```python
from build123d import *

# Parameters (mm, degrees)
BOSS_EXTRUDE1_DEPTH = 4.4
SKETCH2_R           = 9.375
BOSS_EXTRUDE2_DEPTH = 0.9
SKETCH3_R           = 7
BOSS_EXTRUDE3_DEPTH = 0.1
SKETCH4_R           = 2.8
BOSS_EXTRUDE4_DEPTH = 2.5
SKETCH5_R           = 5.5
BOSS_EXTRUDE5_DEPTH = 1.5
FILLET1_R           = 1
BOSS_EXTRUDE6_START = -0.8
BOSS_EXTRUDE6_DEPTH = 1.2
SKETCH7_R           = 1
BOSS_EXTRUDE7_DEPTH = 1.2


with BuildPart() as part:
    # Sketch1 → Boss-Extrude1 (new body)
    with BuildSketch(Plane(origin=(-40.787368979, -82.87971859, -2.365032328), x_dir=(1, 0, 0), z_dir=(0, 1, 0))):
        Polygon((28.025105958, 37.98255848), (31.581105958, 34.42655848), (31.581105958, 22.78855848), (28.025105958, 19.23255848), (16.387105958, 19.23255848), (12.831105958, 22.78855848), (12.831105958, 34.42655848), (16.387105958, 37.98255848), align=None)
    extrude(amount=BOSS_EXTRUDE1_DEPTH)

    # Sketch2 → Boss-Extrude2 (add)
    with BuildSketch(Plane(origin=(0, -78.47971859, 0), x_dir=(1, 0, 0), z_dir=(0, 1, 0))):
        with Locations(Location((-18.581263021, 30.972590809, 0), (0, 0, 270))):
            Circle(SKETCH2_R)
    extrude(amount=BOSS_EXTRUDE2_DEPTH)

    # Sketch3 → Boss-Extrude3 (add)
    with BuildSketch(Plane(origin=(0, -77.57971859, 0), x_dir=(1, 0, 0), z_dir=(0, 1, 0))):
        with Locations(Location((-18.581263021, 30.972590809, 0), (0, 0, 270))):
            Circle(SKETCH3_R)
    extrude(amount=BOSS_EXTRUDE3_DEPTH)

    # Sketch4 → Boss-Extrude4 (add)
    with BuildSketch(Plane(origin=(0, -77.47971859, 0), x_dir=(1, 0, 0), z_dir=(0, 1, 0))):
        with Locations(Location((-18.581263021, 30.972590809, 0), (0, 0, 270))):
            Circle(SKETCH4_R)
    extrude(amount=BOSS_EXTRUDE4_DEPTH)

    # Sketch5 → Boss-Extrude5 (add)
    with BuildSketch(Plane(origin=(0, -74.97971859, 0), x_dir=(1, 0, 0), z_dir=(0, 1, 0))):
        with Locations(Location((-18.581263021, 30.972590809, 0), (0, 0, 270))):
            Circle(SKETCH5_R)
    extrude(amount=BOSS_EXTRUDE5_DEPTH)

    # Fillet1
    fillet1_edges = [part.edges().sort_by_distance(p)[0] for p in [
        (-18.581263021, -73.47971859, -36.472590809),
    ]]
    fillet(fillet1_edges, radius=FILLET1_R)

    # Sketch6 → Boss-Extrude6 (add)
    with BuildSketch(Plane.XZ.offset(82.87971859).offset(BOSS_EXTRUDE6_START)):
        with BuildLine():
            ThreePointArc((-6.691791307, -21.597590809), (-8.244016355, -19.274521857), (-10.984263021, -19.819590809))
            Line((-10.984263021, -19.819590809), (-9.913369802, -20.890484027))
            ThreePointArc((-9.913369802, -20.890484027), (-8.823579589, -20.673711276), (-8.206263021, -21.597590809))
            ThreePointArc((-8.206263021, -21.597590809), (-8.282383489, -21.980274241), (-8.49915624, -22.30469759))
            Line((-8.49915624, -22.30469759), (-7.428263021, -23.375590809))
            ThreePointArc((-7.428263021, -23.375590809), (-6.88319407, -22.559837475), (-6.691791307, -21.597590809))
        make_face()
        with BuildLine():
            Line((-9.913369802, -20.890484027), (-10.984263021, -19.819590809))
            ThreePointArc((-10.984263021, -19.819590809), (-11.720734735, -21.597590809), (-10.984263021, -23.375590809))
            ThreePointArc((-10.984263021, -23.375590809), (-9.206263021, -24.112062522), (-7.428263021, -23.375590809))
            Line((-7.428263021, -23.375590809), (-8.49915624, -22.30469759))
            ThreePointArc((-8.49915624, -22.30469759), (-9.913369802, -22.30469759), (-9.913369802, -20.890484027))
        make_face()
        with BuildLine():
            Line((-10.984263021, -19.819590809), (-12.762263021, -21.597590809))
            Line((-12.762263021, -21.597590809), (-10.984263021, -23.375590809))
            ThreePointArc((-10.984263021, -23.375590809), (-11.720734735, -21.597590809), (-10.984263021, -19.819590809))
        make_face()
        with BuildLine():
            ThreePointArc((-7.428263021, -23.375590809), (-9.206263021, -24.112062522), (-10.984263021, -23.375590809))
            Line((-10.984263021, -23.375590809), (-9.206263021, -25.153590809))
            Line((-9.206263021, -25.153590809), (-7.428263021, -23.375590809))
        make_face()
    extrude(amount=-BOSS_EXTRUDE6_DEPTH)

    # Sketch7 → Boss-Extrude7 (add)
    with BuildSketch(Plane.XZ.offset(82.07971859)):
        with BuildLine():
            Line((-9.206263021, -36.791590809), (-9.206263021, -42.347590809))
            ThreePointArc((-9.206263021, -42.347590809), (-9.49915624, -43.05469759), (-10.206263021, -43.347590809))
            Line((-10.206263021, -43.347590809), (-11.762263021, -43.347590809))
            ThreePointArc((-11.762263021, -43.347590809), (-12.469369802, -43.05469759), (-12.762263021, -42.347590809))
            Line((-12.762263021, -42.347590809), (-12.762263021, -40.347590809))
            Line((-12.762263021, -40.347590809), (-9.206263021, -36.791590809))
        make_face()
        with Locations(Location((-10.984263021, -41.347590809, 0), (0, 0, 270))):
            Circle(SKETCH7_R, mode=Mode.SUBTRACT)
    extrude(amount=-BOSS_EXTRUDE7_DEPTH)


solid = part.part
```
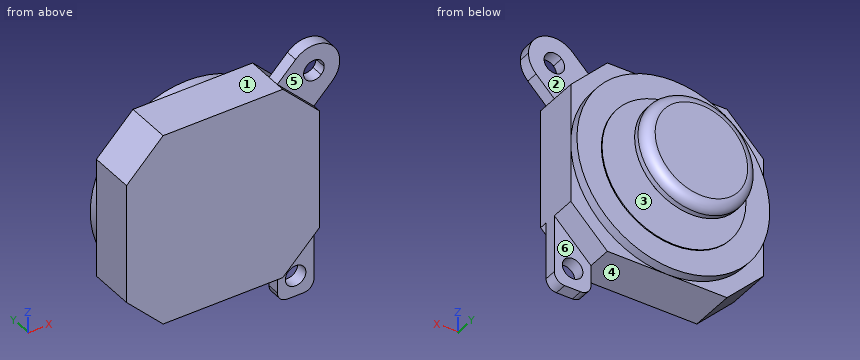
Work out the finished part from the listing and answer in its coordinate system (mm). Face numbers are marked on the shaded views. A direction names the side the tool comes from. Give positions to 0.01 mm unless a question says otherwise; leave off trailing zeros. Write each loop counter-clockwise with the first axis right and the second up, starting at its lowest first coordinate (ties: lowest second). Pieces come first, ordered by that corner, then holes. Notation, with made-up numbers: (37.25, 12) - (66.25, 12) arc R26 ccw to (66.25, 36) - close; hole circle Ø4 at (-27.5, -19). An arc over 180 degrees is marked (long way). Use one line per item in the form item = value.
1. Consider L1, parallel to Y at x = -26.75, z = -33.5; L2, parallel to X at y = -80.25, z = -26; L3, parallel to Y at x = -11.75, z = -24.5. Determine where each line is inside the solid, lowest interval first.
Filled in:
L1 = -82.88 to -77.58
L2 = -27.96 to -9.21
L3 = -82.88 to -78.48
2. A cutting plane is placed at A-A (y = -80.25). Write down the section's boundary in (x, z), and give its area (3 significant figures).
Filled in:
outline = (-27.96, -36.79) - (-24.4, -40.35) - (-12.76, -40.35) - (-9.21, -36.79) - (-9.21, -25.15) - (-12.76, -21.6) - (-24.4, -21.6) - (-27.96, -25.15) - close
area = 326 mm^2
3. For the marked faces 4, 5 and 6, determine the directions among +Z, -Z, +X, -X, +Y, -Y from which every point of the face is accessible in a straight line to the end or side of a thin tool.
Filled in:
face_4 = -Z, -X, +Y, -Y
face_5 = +Z, +X, -Y
face_6 = -Z, +X, +Y
4. Each of these flat-tipped pins is pushed along its axis until it touches: pin 1 Ø1.8 at (x, z) = (-10.5, -39) entering from +Y; pin 2 Ø3 at (x, z) = (-21, -25) entering from +Y; pin 3 Ø5 at (x, z) = (-9, -21) entering from +Y. Where does it stop, or does it pass through?
Filled in:
pin_1 = -78.48
pin_2 = -73.58
pin_3 = -80.88
5. A cutting plane is placed at C-C (y = -76). Write down the section's boundary in (x, z).
Filled in:
outline = circle Ø5.6 at (-18.58, -30.97)
6. Determine the mould class of the marked faces 1, 2 and 3 for opening direction Y: released by +Y, released by -Y, zero draft, split by the parting line, or undercut.
Filled in:
face_1 = zero draft
face_2 = released by +Y
face_3 = undercut
7. A cutting plane is placed at B-B (z = -41.5). Write down the section's boundary in (x, y), and give its area (3 significant figures).
Filled in:
outline = (-12.76, -82.08) - (-11.97, -82.08) - (-11.97, -80.88) - (-12.76, -80.88) - close; (-10, -82.08) - (-9.21, -82.08) - (-9.21, -80.88) - (-10, -80.88) - close
area = 1.90 mm^2
